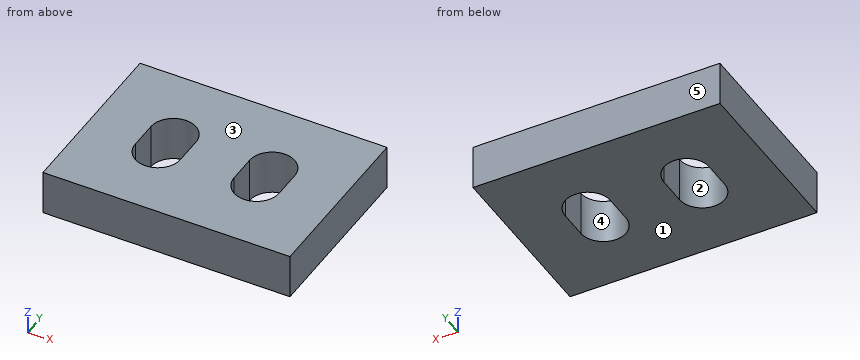
Autodesk Inventor part; units mm, degrees
ref_plane "YZ Plane" through (0, 0, 0) normal (1, 0, 0) x (0, 1, 0)
ref_plane "XZ Plane" through (0, 0, 0) normal (0, 1, 0) x (-1, 0, 0)
ref_plane "XY Plane" through (0, 0, 0) normal (0, 0, 1) x (1, 0, 0)
sketch "Sketch1" plane through (0, 0, 0) normal (0, 0, 1) x (1, 0, 0)
  line L0 (0, 0) -> (0, 12.5)
  line L1 (0, 12.5) -> (8.75, 12.5)
  line L2 (8.75, 12.5) -> (8.75, 0)
  line L3 (8.75, 0) -> (0, 0)
  line L4 (3.5, 7.25) -> (3.5, 5.25) construction
  line L5 (1.9, 7.25) -> (1.9, 5.25)
  line L6 (5.1, 5.25) -> (5.1, 7.25)
  arc A0 (5.1, 7.25) -> (1.9, 7.25) centre (3.5, 7.25) ccw
  arc A1 (1.9, 5.25) -> (5.1, 5.25) centre (3.5, 5.25) ccw
  point P0 (3.5, 6.25)
  dimension "d13" = 3.2
  dimension "d14" = 2
  dimension "d15" = 6.25
  dimension "d17" = 12.5
  dimension "d18" = 8.75
  dimension "d19" = 3.5
extrude "Extrusion1" add sketch "Sketch1" along normal blind 3.175
mirror "Mirror1" about plane through (0, 12.5, 0) normal (-1, 0, 0) of "Extrusion1"
equation "\"d8\" = THICKA"
equation "\"THICKA\" = 3.175"
equation "\"THICKB\" = 6.731"
equation "\"THICKC\" = 12.7"
equation "\"MAGDIA\" = 9.5"
equation "\"BALLDIA\" = 12"
properties part number "Air2D_Hinge_Top"
The model under review builds one solid part; all positions refer to its coordinate system, in mm. Face numbers are marked on the shaded views. A direction names the side the tool comes from. Round coordinates to 2 decimals unless told otherwise and drop trailing zeros. Loops run counter-clockwise (first coordinate to the right, second up) from the corner with the lowest first, then second, coordinate; pieces in that order, holes last. Notation, with made-up numbers: M 65.25,-4.5 L 85.25,-4.5 A33 cw 85.25,24.5 Z; hole C -36.5,78 d7. An arc over 180 degrees is marked long. Answer as CSV lines item,"result". Start each with the question number.
Item 1: Consider section C-C (y = 8.5). Write out the cut boundary in (x, z) (3 decimals), then the cut area to 3 significant figures.
Item 2: Mouldability with a two-part tool opening along Y and no side actions: class the marked faces 3, 4 and 5 as released by +Y, released by -Y, zero draft, split by the parting line, or undercut.
Item 3: Consider section A-A (x = 3.5). Write out the cut boundary in (y, z) (3 decimals).
Item 4: For the marked faces 1 and 2, list the 3-axis set-ups (+Z, -Z, +X, -X, +Y, -Y) from which the entire face can be reached by the end or side of a thin tool; tool diameter is ignored.
Item 5: Wall thickness on line 1 (X direction, y = 6, z = 1.8); line 2 (Y direction, x = 3.5, z = 0.3); line 3 (X direction, y = 4.25, z = 1.85): over which ranges is each line inside the solid? List them lowest first. Write a range as [from, to].
Item 6: Consider section B-B (z = 0.7). Write out the cut boundary in (x, y), then the cut area to 3 significant figures.
Answer:
1,outline,"M -8.75,0 L -4.499,0 L -4.499,3.175 L -8.75,3.175 Z; M -2.501,0 L 2.501,0 L 2.501,3.175 L -2.501,3.175 Z; M 4.499,0 L 8.75,0 L 8.75,3.175 L 4.499,3.175 Z"
1,area,"42.9 mm^2"
2,face 3,"zero draft"
2,face 4,"undercut"
2,face 5,"released by +Y"
3,outline,"M 0,0 L 3.65,0 L 3.65,3.175 L 0,3.175 Z; M 8.85,0 L 12.5,0 L 12.5,3.175 L 8.85,3.175 Z"
4,face 1,"-Z, +X, -X, +Y, -Y"
4,face 2,"+Z, -Z"
5,line 1,"x = [-8.75, -5.1], [-1.9, 1.9], [5.1, 8.75]"
5,line 2,"y = [0, 3.65], [8.85, 12.5]"
5,line 3,"x = [-8.75, -4.75], [-2.25, 2.25], [4.75, 8.75]"
6,outline,"M -8.75,0 L 8.75,0 L 8.75,12.5 L -8.75,12.5 Z; hole M -5.1,5.25 A1.6 ccw -1.9,5.25 L -1.9,7.25 A1.6 ccw -5.1,7.25 Z; hole M 1.9,5.25 A1.6 ccw 5.1,5.25 L 5.1,7.25 A1.6 ccw 1.9,7.25 Z"
6,area,"190 mm^2"
